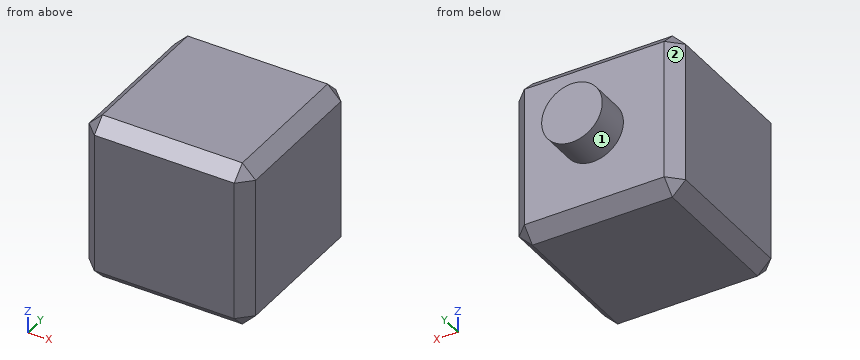
from build123d import *

# Parameters (mm, degrees)
F0_W     = 63.5
F0_H     = 63.5
F1_DEPTH = 63.5
F2_SIZE  = 5.08
F3_R     = 11.556322
F4_DEPTH = 76.708


with BuildPart() as f1:
    # F0 (on Front) → F1 (new body)
    with BuildSketch(Plane.XZ):
        with Locations((-4.667691, -2.960291)):
            Rectangle(F0_W, F0_H)
    extrude(amount=-F1_DEPTH)

    # F2
    f2_edges = [f1.edges().sort_by_distance(p)[0] for p in [
        (-4.667691, 0, 28.789709),
        (27.082309, 31.75, 28.789709),
        (-36.417691, 31.75, 28.789709),
        (-4.667691, 63.5, 28.789709),
        (27.082309, 0, -2.960291),
        (27.082309, 63.5, -2.960291),
        (-36.417691, 0, -2.960291),
        (-36.417691, 63.5, -2.960291),
        (-4.667691, 63.5, -34.710291),
        (27.082309, 31.75, -34.710291),
        (-4.667691, 0, -34.710291),
        (-36.417691, 31.75, -34.710291),
    ]]
    chamfer(f2_edges, length=F2_SIZE)

    # F3 (on face) → F4 (join)
    with BuildSketch(Plane.XZ):
        with Locations((-4.20644, -2.541391)):
            Circle(F3_R)
    extrude(amount=-F4_DEPTH)


solid = f1.part
The listing builds one solid part. Answer for the finished solid, in the listing's coordinates (mm). Face numbers are marked on the shaded views. A direction names the side the tool comes from. Give positions to 0.01 mm unless a question says otherwise; leave off trailing zeros. Order: outer loops, then holes, each group sorted by start corner. A loop starts at its lowest first (then second) coordinate and runs counter-clockwise, first axis right, second up. Notation, with made-up numbers: (20.5, 11.5) - (72.5, 11.5) arc R38 ccw to (72.5, 50.5) - close; hole circle Ø9 at (5.25, 51). An arc over 180 degrees is marked (long way). One line per item, written item: value. Start each with the question number.
1) A cutting plane is placed at A-A on z = -28.5. Give the vertices of the cut face in (x, y).
2) A cutting plane is placed at D-D on z = 7. Give the vertices of the cut face in (x, y), then the cut area to 3 significant figures.
3) A cutting plane is placed at B-B on x = 10.5. Give the vertices of the cut face in (y, z), then the cut area to 3 significant figures.
4) Given pin 1 Ø6 at (y, z) = (66, -2) entering from -X; pin 2 Ø1 at (x, z) = (-12, -13) entering from +Y, each flat-ended and moving along its own axis, determine where each tip first touches the part or whether it passes through.
5) A cutting plane is placed at C-C on y = 72.5. Give the vertices of the cut face in (x, z).
6) Find the intervals of material crossed by L1, parallel to Y at x = -5, z = -20.5; L2, parallel to X at y = 52, z = 25.5; L3, parallel to X at y = 4, z = 19, in increasing order.
7) A tool of negligible diameter and unlimited length cuts with its end or side. For the marked faces 1 and 2, from which of +Z, -Z, +X, -X, +Y, -Y can it reach the whole face along a straight path? Write none if from no direction.
Answer sheet:
1. outline: (-36.42, 5.08) - (-31.34, 0) - (22, 0) - (27.08, 5.08) - (27.08, 58.42) - (22, 63.5) - (-31.34, 63.5) - (-36.42, 58.42) - close
2. outline: (-36.42, 5.08) - (-31.34, 0) - (22, 0) - (27.08, 5.08) - (27.08, 58.42) - (22, 63.5) - (2.31, 63.5) - (2.31, 76.71) - (-10.73, 76.71) - (-10.73, 63.5) - (-31.34, 63.5) - (-36.42, 58.42) - close
2. area: 4,150 mm2
3. outline: (0, -29.63) - (5.08, -34.71) - (58.42, -34.71) - (63.5, -29.63) - (63.5, 23.71) - (58.42, 28.79) - (5.08, 28.79) - (0, 23.71) - close
3. area: 3,980 mm2
4. pin 1: stops at x = -31.84
4. pin 2: stops at y = 63.5
5. outline: circle Ø23.11 at (-4.21, -2.54)
6. L1: y = 0 to 63.5
6. L2: x = -34.63 to 25.29
6. L3: x = -35.34 to 26
7. face 1: +Y
7. face 2: +Z, -Z, -X, +Y
